Design review of the part built by this model. Coordinates are the model's own, in mm. A direction names the side the tool comes from. Round coordinates to 2 decimals unless told otherwise and drop trailing zeros. Write each loop counter-clockwise with the first axis right and the second up, starting at its lowest first coordinate (ties: lowest second). Pieces come first, ordered by that corner, then holes. Notation, with made-up numbers: (21.25, 27.25) -> (33.25, 27.25) arc R15 ccw to (33.25, 50.25) -> close; hole circle Ø8 at (27, 42). An arc over 180 degrees is marked (long way). One line per question, with ' | ' between items. Start each with the question number.
1) Consider section C-C (z = 19). Give the boundary of the cut face in (x, y) (3 decimals), then the cut area to 3 significant figures.
2) Consider section A-A (y = 0). Give the boundary of the cut face in (x, z) (3 decimals), then the cut area to 3 significant figures.
3) Insertion check: pin 1 Ø2 at (x, z) = (4.5, 42.5) entering from -Y; pin 2 Ø5.5 at (x, z) = (-1.5, 24.5) entering from +Y; pin 3 Ø8 at (x, z) = (-6.5, 35.5) entering from +Y; pin 4 Ø2 at (x, y) = (-2, -6) entering from -Z. Each pin has a flat end and moves straight along its axis. Give the tip position at first contact, or say it passes through.
4) For probe 1 along Z at (x, y) = (5, 0) (3 decimals); probe 2 along Y at (x, z) = (2.75, 38.1); probe 3 along Y at (x, z) = (4, 38.1), list the stretches that pass through material, from the lowest coordinate up.
5) Mouldability with a two-part tool opening along Z and no side actions: class faces 1 (the flat face through (0, 0, 0)), 2 (the cylindrical face through (0.13, -0.517, 42.035)), 3 (the flat face through (0, 0, 66.675)), 4 (the cylindrical face through (4.4, -8.45, 34.48)) as +Z half, -Z half, draft (parallel to the pull), parting line (faces both ways), or undercut.
6) Consider section D-D (z = 38.1). Give the boundary of the cut face in (x, y) (3 decimals).
7) For faces 5 (the conical face through (-1.41, -6.349, 0.154)), 6 (the flat face through (0, 7.943, 21)), list the 3-axis set-ups (+Z, -Z, +X, -X, +Y, -Y) from which the entire face can be reached by the end or side of a thin tool; tool diameter is ignored.
```python
from build123d import *

# Parameters (mm, degrees)
F0_R     = 9.525
F1_DEPTH = 66.675
F2_SIZE  = 3.175
F3_W     = 33.163304
F3_H     = 21.43125
F3_W_2   = 1.5875
F3_R     = 3.96875
F4_DEPTH = 40.839933


with BuildPart() as f1:
    # F0 (on Top) → F1 (new body)
    with BuildSketch(Plane.XY):
        Circle(F0_R)
    extrude(amount=F1_DEPTH)

    # F2
    f2_edges = [f1.edges().sort_by_distance(p)[0] for p in [
        (-9.525, 0, 0),
    ]]
    chamfer(f2_edges, length=F2_SIZE)

    # F3 (on Right) → F4 (cut, symmetric)
    with BuildSketch(Plane.YZ):
        with Locations((26.112016, 21.034375)):
            Rectangle(F3_W, F3_H)
        with Locations((8.736614, 21.034375)):
            Rectangle(F3_W_2, F3_H)
        with Locations((0, 38.1)):
            Circle(F3_R)
    extrude(amount=F4_DEPTH, both=True, mode=Mode.SUBTRACT)


solid = f1.part
```
From the geometry:
1) outline: (-5.257, 7.943) arc R9.525 ccw (long way) to (5.257, 7.943) -> close | area: 274 mm2
2) outline: (-9.525, 3.175) -> (-6.35, 0) -> (6.35, 0) -> (9.525, 3.175) -> (9.525, 34.131) -> (-9.525, 34.131) -> close; (-9.525, 42.069) -> (9.525, 42.069) -> (9.525, 66.675) -> (-9.525, 66.675) -> close | area: 1,110 mm2
3) pin 1: stops at y = -8.86 | pin 2: stops at y = 7.94 | pin 3: stops at y = 9.19 | pin 4: stops at z = 0
4) probe 1: z = 0 to 34.131, 42.069 to 66.675 | probe 2: y = -9.12 to -3.97, 3.97 to 9.12 | probe 3: y = -8.64 to -3.97, 3.97 to 8.64
5) face 1: -Z half | face 2: undercut | face 3: +Z half | face 4: draft
6) outline: (-8.659, -3.969) arc R9.525 ccw to (8.659, -3.969) -> close; (-8.659, 3.969) -> (8.659, 3.969) arc R9.525 ccw to start
7) face 5: -Z | face 6: +X, -X, +Y
